Part print with two shaded views. Sizes in mm from the minimum x, y, z corner. A direction names the side the tool comes from. Coordinates: 2 decimals unless noted, no trailing zeros. Loops run counter-clockwise (first coordinate to the right, second up) from the corner with the lowest first, then second, coordinate; pieces in that order, holes last.
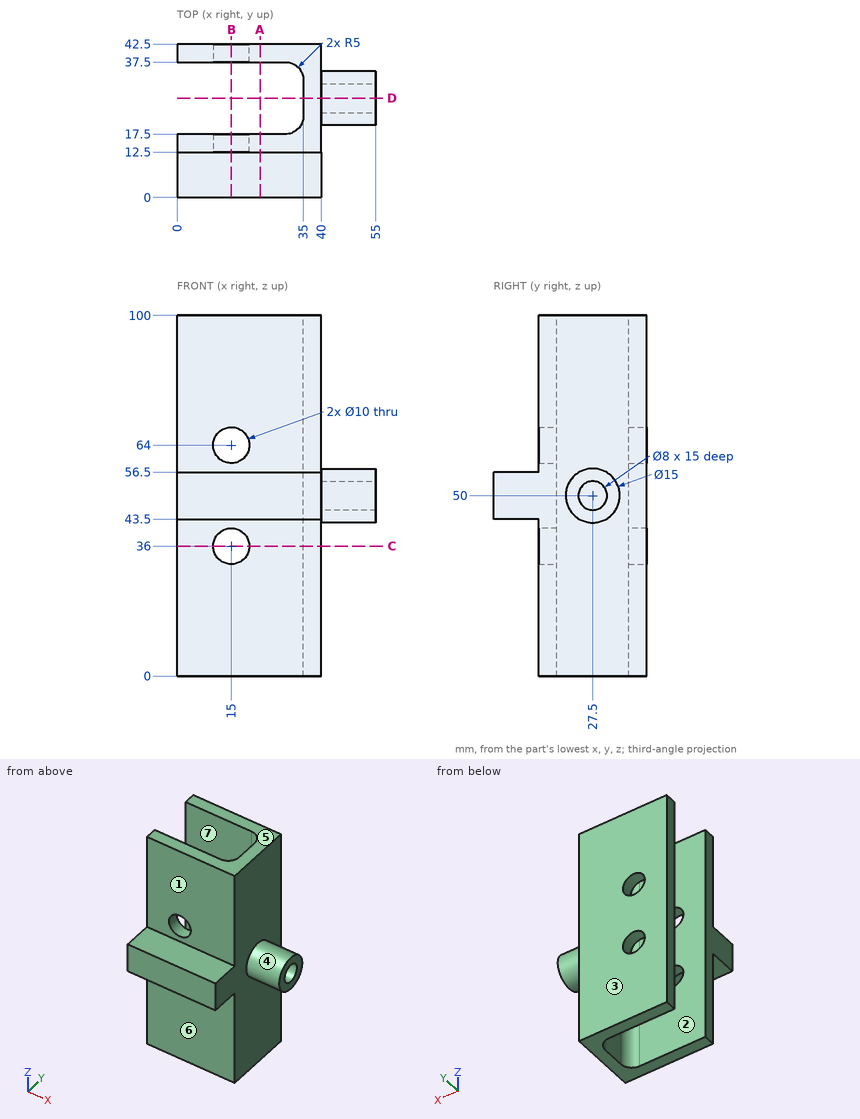
Q1. Slice it at D-D (y = 27.5). List the corners of the cut face in (x, z), and give its area (3 significant figures).
Answers:
outline: (35, 0) - (40, 0) - (40, 42.5) - (55, 42.5) - (55, 46) - (40, 46) - (40, 54) - (55, 54) - (55, 57.5) - (40, 57.5) - (40, 100) - (35, 100) - close
area: 605 mm2
Q2. Which spindle directions (+Z, -Z, +X, -X, +Y, -Y) get a long thin tool onto all of the face, cutting with end or side? Do the marked faces 1, 2, 3 and 4. Say none if no direction does.
Answers:
face 1: +Z, +X, -X, -Y
face 2: +Z, -Z, -X
face 3: +Z, -Z, +X, -X, +Y
face 4: +X
Q3. Mould opens along Y. For the marked faces 5, 6 and 7 say: +Y half, -Y half, draft (parallel to the pull), parting line (faces both ways), or undercut.
Answers:
face 5: draft
face 6: -Y half
face 7: undercut
Q4. Slice it at C-C (z = 36). List the corners of the cut face in (x, y), and give its area (3 significant figures).
Answers:
outline: (0, 12.5) - (10, 12.5) - (10, 17.5) - (0, 17.5) - close; (0, 37.5) - (10, 37.5) - (10, 42.5) - (0, 42.5) - close; (20, 12.5) - (40, 12.5) - (40, 42.5) - (20, 42.5) - (20, 37.5) - (30, 37.5) arc R5 cw to (35, 32.5) - (35, 22.5) arc R5 cw to (30, 17.5) - (20, 17.5) - close
area: 411 mm2
Q5. Slice it at A-A (x = 23). List the corners of the cut face in (y, z), and give its area (3 significant figures).
Answers:
outline: (0, 43.5) - (12.5, 43.5) - (12.5, 0) - (17.5, 0) - (17.5, 100) - (12.5, 100) - (12.5, 56.5) - (0, 56.5) - close; (37.5, 0) - (42.5, 0) - (42.5, 100) - (37.5, 100) - close
area: 1,160 mm2
Q6. Drill centre lines: line 1 (Y direction, x = 21, z = 12.5); line 2 (Y direction, x = 52, z = 50); line 3 (Y direction, x = 39.5, z = 31). Where is each one in solid material? Low to high.
Answers:
line 1: y = 12.5 to 17.5, 37.5 to 42.5
line 2: y = 20 to 23.5, 31.5 to 35
line 3: y = 12.5 to 42.5
Q7. Flat gauge pins, fed straight in: P1, Ø2.5, axis at y = 26.5, z = 50.5, coming from the +X side; P2, Ø3, axis at y = 35, z = 10, coming from the -X side; P3, Ø20, axis at x = 18.5, z = 30.5, coming from the -Y side. Where does each tip first touch, or does it go through?
Answers:
P1: stops at x = 40
P2: stops at x = 33
P3: stops at y = 12.5
Q8. Slice it at B-B (x = 15). List the corners of the cut face in (y, z).
Answers:
outline: (0, 43.5) - (12.5, 43.5) - (12.5, 41) - (17.5, 41) - (17.5, 59) - (12.5, 59) - (12.5, 56.5) - (0, 56.5) - close; (12.5, 0) - (17.5, 0) - (17.5, 31) - (12.5, 31) - close; (12.5, 69) - (17.5, 69) - (17.5, 100) - (12.5, 100) - close; (37.5, 0) - (42.5, 0) - (42.5, 31) - (37.5, 31) - close; (37.5, 41) - (42.5, 41) - (42.5, 59) - (37.5, 59) - close; (37.5, 69) - (42.5, 69) - (42.5, 100) - (37.5, 100) - close
